from build123d import *

# Parameters (mm, degrees)
SKETCH005_W            = 259.2
SKETCH005_H            = 259.2
PAD003_DEPTH           = 3
SKETCH006_W            = 215.2
SKETCH006_H            = 11
POCKET002_DEPTH        = 3.001
LINEARPATTERN004_COUNT = 12
LINEARPATTERN004_PITCH = 16.6
SKETCH009_W            = 10
SKETCH009_H            = 27.6
POCKET004_DEPTH        = 742.153863
LINEARPATTERN006_COUNT = 6
LINEARPATTERN006_PITCH = 33.2
SKETCH010_W            = 10
SKETCH010_H            = 27.6
POCKET005_DEPTH        = 9.001
LINEARPATTERN007_COUNT = 5
LINEARPATTERN007_PITCH = 33.2
SKETCH012_R            = 3
POCKET007_DEPTH        = 9.001


with BuildPart() as part:
    # Sketch005 → Pad003 (new body)
    with BuildSketch(Plane.XY.offset(-6)):
        Rectangle(SKETCH005_W, SKETCH005_H)
    extrude(amount=-PAD003_DEPTH)

    # Sketch006 (on Face6 of Pad003) → Pocket002 (cut, through all)
    with BuildSketch(Plane(origin=(0, 0, -9), x_dir=(1, 0, 0), z_dir=(0, 0, -1))):
        with Locations((0, 91.3)):
            Rectangle(SKETCH006_W, SKETCH006_H)
    pocket002 = extrude(amount=-POCKET002_DEPTH, mode=Mode.SUBTRACT)

    # LinearPattern004: Pocket002 ×12
    with Locations(*[(0, i * LINEARPATTERN004_PITCH, 0) for i in range(1, LINEARPATTERN004_COUNT)]):
        add(pocket002, mode=Mode.SUBTRACT)

    # Sketch009 → Pocket004 (cut, through all)
    with BuildSketch(Plane.XY):
        with Locations((102.6, 83)):
            Rectangle(SKETCH009_W, SKETCH009_H)
    pocket004 = extrude(amount=-POCKET004_DEPTH, mode=Mode.SUBTRACT)

    # LinearPattern006: Pocket004 ×6
    with Locations(*[(0, -i * LINEARPATTERN006_PITCH, 0) for i in range(1, LINEARPATTERN006_COUNT)]):
        add(pocket004, mode=Mode.SUBTRACT)

    # Sketch010 → Pocket005 (cut, through all)
    with BuildSketch(Plane.XY):
        with Locations((-102.6, 66.4)):
            Rectangle(SKETCH010_W, SKETCH010_H)
    pocket005 = extrude(amount=-POCKET005_DEPTH, mode=Mode.SUBTRACT)

    # LinearPattern007: Pocket005 ×5
    with Locations(*[(0, -i * LINEARPATTERN007_PITCH, 0) for i in range(1, LINEARPATTERN007_COUNT)]):
        add(pocket005, mode=Mode.SUBTRACT)

    # Sketch012 → Pocket007 (cut, through all)
    with BuildSketch(Plane.XY):
        with Locations((-112.5, 112.5)):
            Circle(SKETCH012_R)
        with Locations((112.5, 112.5)):
            Circle(SKETCH012_R)
        with Locations((112.5, -112.5)):
            Circle(SKETCH012_R)
        with Locations((-112.5, -112.5)):
            Circle(SKETCH012_R)
    extrude(amount=-POCKET007_DEPTH, mode=Mode.SUBTRACT)


solid = part.part
Verification items for the finished model (mm, model axes). Coordinates: 2 decimals unless noted, no trailing zeros. Order: outer loops, then holes, each group sorted by start corner. A loop starts at its lowest first (then second) coordinate and runs counter-clockwise, first axis right, second up. Notation, with made-up numbers: M 16,69 L 35,69 A21 ccw 35,81 Z; hole C -1.5,56 d4. An arc over 180 degrees is marked long. One line per item, written item: value. Start each with the question number.
Item 1: Sectioned sample at C-C on z = -8.3. Give the number of separate pieces and of enclosed holes in the cut face, then the cut area to 3 significant figures.
Item 2: Sectioned sample at B-B on y = 60. Record the cut outline in (x, z), then the cut area to 3 significant figures.
Item 3: Depth check by flat-ended pin: P1, Ø4, axis at x = 48.5, y = 22, coming from the -Z side. Enter the tip coordinate at first touch or a pass-through.
Item 4: Sectioned sample at A-A on x = 112.5. Record the cut outline in (y, z).
Item 5: Mould release check, pull along Y, two halves, no side actions. Record for faces 1 (the cylindrical face through (115.36, -111.6, -7.48)), 2 (the cylindrical face through (-109.64, 113.4, -7.48)), 3 (the flat face through (-2, 2, -6)): pulls with the +Y half, pulls with the -Y half, needs draft (parallel to the pull), parting line crosses it, or undercut.
Item 6: Thickness scan on probe 1 along Y at (x, z) = (112.5, -8); probe 2 along X at (y, z) = (-33, -8.65); probe 3 along X at (y, z) = (-37.5, -7). Record the ranges inside material, lowest first.
Calculated:
1. separate pieces: 1
1. enclosed holes: 5
1. area: 38,000 mm^2
2. outline: M -129.6,-9 L -107.6,-9 L -107.6,-6 L -129.6,-6 Z; M 107.6,-9 L 129.6,-9 L 129.6,-6 L 107.6,-6 Z
2. area: 132 mm^2
3. P1: through
4. outline: M -129.6,-9 L -115.5,-9 L -115.5,-6 L -129.6,-6 Z; M -109.5,-9 L 109.5,-9 L 109.5,-6 L -109.5,-6 Z; M 115.5,-9 L 129.6,-9 L 129.6,-6 L 115.5,-6 Z
5. face 1: undercut
5. face 2: undercut
5. face 3: needs draft
6. probe 1: -129.6 to -115.5, -109.5 to 109.5, 115.5 to 129.6
6. probe 2: -129.6 to -107.6, -97.6 to 129.6
6. probe 3: -129.6 to -107.6, 107.6 to 129.6
